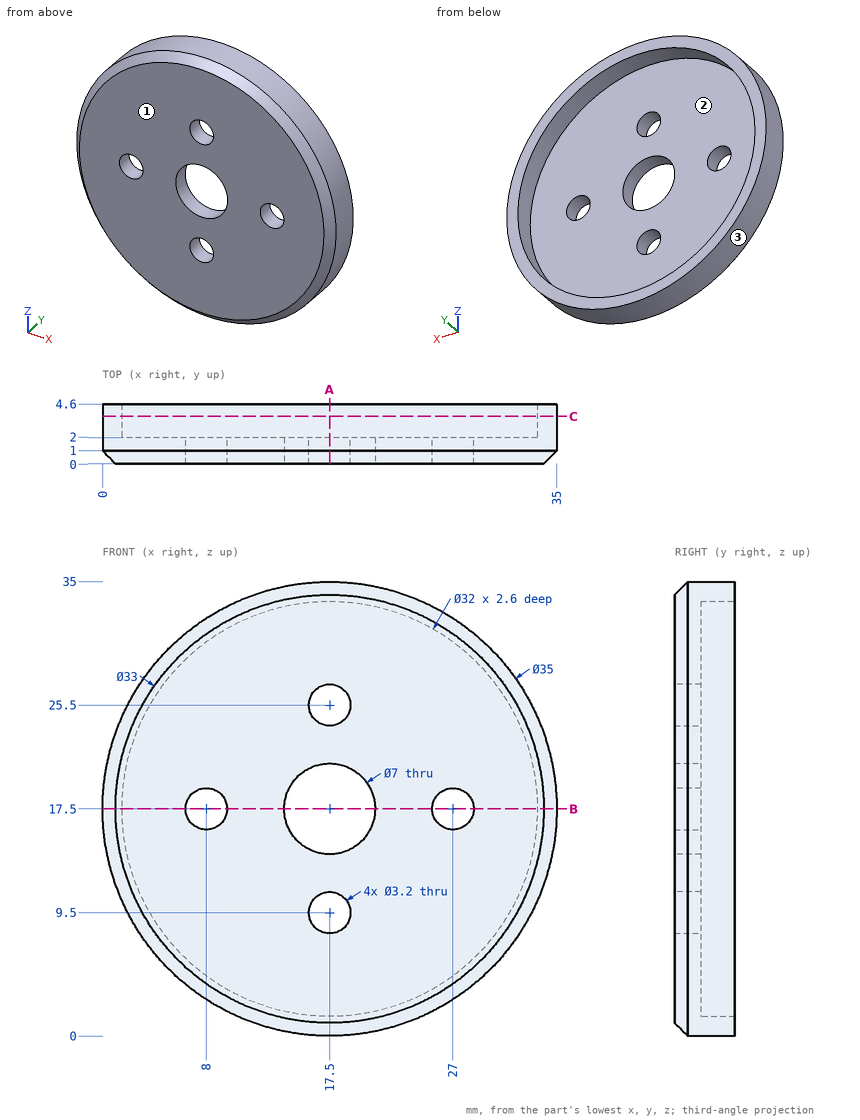
Job drawing, mm, ordinate dimensions from the low corner. One solid piece. Give positions to 0.01 mm unless a question says otherwise; leave off trailing zeros. Order: outer loops, then holes, each group sorted by start corner. A loop starts at its lowest first (then second) coordinate and runs counter-clockwise, first axis right, second up. Notation, with made-up numbers: (30, 19.5) - (81, 19.5) arc R26 cw to (81, 45.5) - close; hole circle Ø9 at (-28, 30). An arc over 180 degrees is marked (long way). One line per question, with ' | ' between items.
1. Band-saw the part on C-C on y = 3.65. List the corners of the cut face in (x, z), then the cut area to 3 significant figures.
Filled in:
outline: circle Ø35 at (17.5, 17.5); hole circle Ø32 at (17.5, 17.5) | area: 158 mm²
2. Band-saw the part on B-B on z = 17.5. List the corners of the cut face in (x, y), then the cut area to 3 significant figures.
Filled in:
outline: (0, 1) - (1, 0) - (6.4, 0) - (6.4, 2) - (1.5, 2) - (1.5, 4.6) - (0, 4.6) - close; (9.6, 0) - (14, 0) - (14, 2) - (9.6, 2) - close; (21, 0) - (25.4, 0) - (25.4, 2) - (21, 2) - close; (28.6, 0) - (34, 0) - (35, 1) - (35, 4.6) - (33.5, 4.6) - (33.5, 2) - (28.6, 2) - close | area: 50.0 mm²
3. Drop a flat-ended pin along its axis: P1, Ø4, axis at x = 17.5, z = 25.5, coming from the +Y side. Give the stop position or say it passes through.
Filled in:
P1: y = 2
4. Band-saw the part on A-A on x = 17.5. List the corners of the cut face in (y, z).
Filled in:
outline: (0, 1) - (1, 0) - (4.6, 0) - (4.6, 1.5) - (2, 1.5) - (2, 7.9) - (0, 7.9) - close; (0, 11.1) - (2, 11.1) - (2, 14) - (0, 14) - close; (0, 21) - (2, 21) - (2, 23.9) - (0, 23.9) - close; (0, 27.1) - (2, 27.1) - (2, 33.5) - (4.6, 33.5) - (4.6, 35) - (1, 35) - (0, 34) - close
5. Drill centre lines: probe 1 along X at (y, z) = (1.05, 17.5); probe 2 along Y at (x, z) = (21, 3); probe 3 along Z at (x, y) = (9, 0.75). Where is each one in solid material? Low to high.
Filled in:
probe 1: 0 to 6.4, 9.6 to 14, 21 to 25.4, 28.6 to 35 | probe 2: 0 to 2 | probe 3: 2.49 to 16.25, 18.75 to 32.51
6. Pull direction X, two halves, no side cores. Call the marked faces 1, 2 and 3: +X half, -X half, draft (parallel to the pull), parting line (faces both ways), or undercut.
Filled in:
face 1: draft | face 2: undercut | face 3: parting line
